Verification items for the finished model (mm, model axes). Give positions to 0.01 mm unless a question says otherwise; leave off trailing zeros. Order: outer loops, then holes, each group sorted by start corner. A loop starts at its lowest first (then second) coordinate and runs counter-clockwise, first axis right, second up.
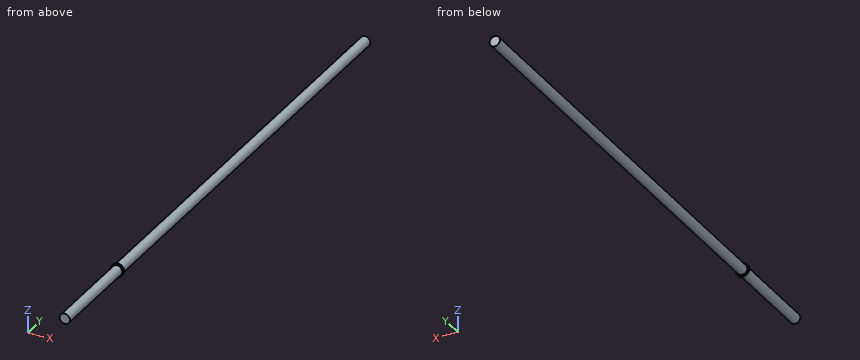
from build123d import *

# Parameters (mm, degrees)
ESBO_O1_R                = 4
RESSALTO_EXTRUS_O2_DEPTH = 445.1
ESBO_O2_W                = 5
ESBO_O2_H                = 1


with BuildPart() as part:
    # Esboço1 → Ressalto-extrusão2 (new body)
    with BuildSketch(Plane(origin=(0, 0, 0), x_dir=(1, 0, 0), z_dir=(0, 1, 0))):
        with Locations(Location((0, 0, 0), (0, 0, 270))):
            Circle(ESBO_O1_R)
    extrude(amount=RESSALTO_EXTRUS_O2_DEPTH)

    # Esboço2 → Revolução1 (revolve)
    with BuildSketch(Plane.XY, mode=Mode.PRIVATE) as revolu_o1_sk:
        with Locations((2.5, 78.05)):
            Rectangle(ESBO_O2_W, ESBO_O2_H)
    revolve(revolu_o1_sk.sketch.rotate(Axis((0, 77.55, 0), (0, 1, 0)), 90), axis=Axis((0, 77.55, 0), (0, 1, 0)))


solid = part.part
(1) Section check B-B, the plane z = 0. Enter the section's corners in (x, y).
Solved:
outline: (-5, 77.55) - (-4, 77.55) - (-4, 0) - (4, 0) - (4, 77.55) - (5, 77.55) - (5, 78.55) - (4, 78.55) - (4, 445.1) - (-4, 445.1) - (-4, 78.55) - (-5, 78.55) - close
(2) Section check C-C, the plane y = 266.5. Enter the section's corners in (x, z).
Solved:
outline: circle Ø8 at (0, 0)
(3) Go/stop test with flat-tipped pins: pin 1 (2 mm diameter, centred on x = -1.5, y = 81, fed in from -Z); pin 2 (4 mm diameter, centred on y = 319, z = 2.5, fed in from +X); pin 3 (1 mm diameter, centred on x = 1.5, y = 47.5, fed in from -Z). Record where each tip stops, or that it passes through.
Solved:
pin 1: stops at z = -3.97
pin 2: stops at x = 3.97
pin 3: stops at z = -3.87
(4) Scan lines: line 1 (Z direction, x = 0, y = 155); line 2 (Y direction, x = 4, z = 2.5); line 3 (X direction, y = 61, z = 0.5). Record each from-to range of solid material in increasing order.
Solved:
line 1: z = -4 to 4
line 2: y = 77.55 to 78.55
line 3: x = -3.97 to 3.97
(5) Section check A-A, the plane x = 0. Enter the section's corners in (y, z).
Solved:
outline: (0, -4) - (77.55, -4) - (77.55, -5) - (78.55, -5) - (78.55, -4) - (445.1, -4) - (445.1, 4) - (78.55, 4) - (78.55, 5) - (77.55, 5) - (77.55, 4) - (0, 4) - close
